Work out the finished part from the listing and answer in its coordinate system (mm). Face numbers are marked on the shaded views. A direction names the side the tool comes from. Coordinates: 2 decimals unless noted, no trailing zeros. Write each loop counter-clockwise with the first axis right and the second up, starting at its lowest first coordinate (ties: lowest second). Pieces come first, ordered by that corner, then holes. Notation, with made-up numbers: (18.25, 77.25) - (47.25, 77.25) arc R22 cw to (47.25, 88.25) - close; hole circle Ø4 at (22, -20.75). An arc over 180 degrees is marked (long way). One line per item, written item: value.
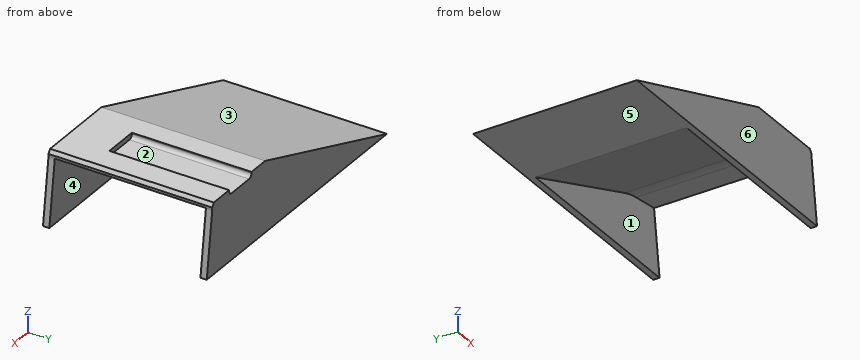
```python
from build123d import *

# Parameters (mm, degrees)
F1_DEPTH      = 6.5
F2_R          = 6
F4_DEPTH      = 0.5
F6_DEPTH      = 3
F6_DEPTH_BACK = 25
F7_SIZE2      = 0.3
F7_SIZE       = 0.2
F8_R          = 0.3


# Not quite as in the source:
# - a pattern or mirror of a feature is missing from the dataset's text; its kind, count and spacing are read off the source's solid


with BuildPart() as f1:
    # F0 (on Front) → F1 (new body, symmetric)
    with BuildSketch(Plane.XZ):
        Polygon((15.2, 5.6), (0, 0), (7, 0), (18.8267862505, 4.7), (21.8, 5.1), (21.8, 5.6), align=None)
    extrude(amount=F1_DEPTH, both=True)

    # F2
    f2_edges = [f1.edges().sort_by_distance(p)[0] for p in [
        (18.826786, 0, 4.7),
    ]]
    fillet(f2_edges, radius=F2_R)

    # F3 (on face) → F4 (join)
    with BuildSketch(Plane(origin=(0, 6.5, 0), x_dir=(-1, 0, 0), z_dir=(0, 1, 0))):
        Polygon((-21.8, 5.6), (-21.8, 5.1), (-22.4861262499, 0), (0, 0), (-15.2, 5.6), align=None)
    f4 = extrude(amount=-F4_DEPTH)

    # F4_copies: F4 across plane
    add(f4.mirror(Plane(origin=(0, 0, 0), x_dir=(0, 0, -1), z_dir=(0, -1, 0))))

    # F5 (on Front) → F6 (cut, two sides)
    with BuildSketch(Plane.XZ) as f6_sk:
        Polygon((18.3, 5.6), (16.9, 5.6), (16.9, 5.2), (19.7, 5.2), (19.7, 5.6), align=None)
    extrude(amount=F6_DEPTH, mode=Mode.SUBTRACT)
    extrude(f6_sk.sketch, amount=-F6_DEPTH_BACK, mode=Mode.SUBTRACT)

    # F7
    f7_edges = [f1.edges().sort_by_distance(p)[0] for p in [
        (21.8, 0, 5.6),
    ]]
    f7_side = f1.faces().sort_by_distance((21.654206, 0, 5.6))[0]
    chamfer(f7_edges, length=F7_SIZE, length2=F7_SIZE2, reference=f7_side)

    # F8
    f8_edges = [f1.edges().sort_by_distance(p)[0] for p in [
        (16.9, 1.75, 5.2),
        (19.7, 1.75, 5.2),
    ]]
    fillet(f8_edges, radius=F8_R)


solid = f1.part
```
Item 1: Consider probe 1 along Y at (x, z) = (21, 3.35); probe 2 along Z at (x, y) = (3.5, -1.75); probe 3 along Z at (x, y) = (5, -5.5). Determine where each line is inside the solid, lowest interval first.
Evaluation:
probe 1: y = -6.5 to -6, 6 to 6.5
probe 2: z = 0 to 1.29
probe 3: z = 0 to 1.84
Item 2: Section B-B, the plane x = 13.5 is taken. Determine the outline of the cut face in (y, z).
Evaluation:
outline: (-6.5, 0) - (-6, 0) - (-6, 2.58) - (6, 2.58) - (6, 0) - (6.5, 0) - (6.5, 4.97) - (-6.5, 4.97) - close
Item 3: Section D-D, the plane x = 6.25 is taken. Determine the outline of the cut face in (y, z), then the cut area to 3 significant figures.
Evaluation:
outline: (-6.5, 0) - (6.5, 0) - (6.5, 2.3) - (-6.5, 2.3) - close
area: 29.9 mm2
Item 4: Which of the six approach directions +Z, -Z, +X, -X, +Y, -Y give full straight-line access (tool end or side, diameter ignored) to the marked faces 1, 2 and 3?
Evaluation:
face 1: -Z, +X
face 2: +Z, +Y
face 3: +Z, -X, +Y, -Y
Item 5: Determine the mould class of the marked faces 4, 5 and 6 for opening direction Y: +Y half, -Y half, draft (parallel to the pull), parting line (faces both ways), or undercut.
Evaluation:
face 4: undercut
face 5: draft
face 6: -Y half
Item 6: Section C-C, the plane z = 1.4 is taken. Determine the outline of the cut face in (x, y).
Evaluation:
outline: (3.8, -6.5) - (22.3, -6.5) - (22.3, -6) - (10.52, -6) - (10.52, 6) - (22.3, 6) - (22.3, 6.5) - (3.8, 6.5) - close
Item 7: Given pin 1 (1.5 mm diameter, centred on x = 18.5, y = -0.5, fed in from -Z); pin 2 (0.7 mm diameter, centred on x = 18, y = 2.5, fed in from +Z); pin 3 (1.5 mm diameter, centred on x = 7, z = 4, fed in from -Y), each flat-ended and moving along its own axis, determine where each tip first touches the part or whether it passes through.
Evaluation:
pin 1: stops at z = 4.27
pin 2: stops at z = 5.2
pin 3: passes through
Item 8: Section A-A, the plane y = -2.75 is taken. Determine the outline of the cut face in (x, z), then the cut area to 3 significant figures.
Evaluation:
outline: (0, 0) - (7, 0) - (18.14, 4.43) arc R6 cw to (19.56, 4.8) - (21.8, 5.1) - (21.8, 5.3) - (21.6, 5.6) - (19.7, 5.6) - (19.7, 5.5) arc R0.3 cw to (19.4, 5.2) - (17.2, 5.2) arc R0.3 cw to (16.9, 5.5) - (16.9, 5.6) - (15.2, 5.6) - close
area: 36.1 mm2
